Read the model definition and answer for the solid it produces. Units are mm, in the model's axes. A direction names the side the tool comes from. Coordinates: 2 decimals unless noted, no trailing zeros. Loops run counter-clockwise (first coordinate to the right, second up) from the corner with the lowest first, then second, coordinate; pieces in that order, holes last. Notation, with made-up numbers: M 21,65.5 L 59,65.5 A25 cw 59,91.5 Z; hole C 54,59 d3. An arc over 180 degrees is marked long. One line per item, written item: value. Start each with the question number.
1. Determine the mould class of faces 1 (the face through (-6, -29.725, -89)), 2 (the face through (-4, 30, -89)), 3 (the face through (-2, -35.725, -89)) for opening direction Y: +Y half, -Y half, draft (parallel to the pull), parting line (faces both ways), or undercut.
2. The part is cut by section A-A (z = -16). Write down the section's boundary in (x, y) (3 decimals).
3. Flat-ended cylindrical pins translate along their axes: pin 1 (1.5 mm diameter, centred on x = 6.5, z = -23, fed in from -Y) (3 decimals); pin 2 (1.2 mm diameter, centred on x = -5, z = -72.5, fed in from +Y) (3 decimals); pin 3 (6.5 mm diameter, centred on y = -26, z = -47.5, fed in from -X). Find the tip coordinate at first contact, or state that the pin passes through.
4. For faces 4 (the face through (-8, -33, -89)), 5 (the face through (8, 23.725, -89)), 6 (the face through (-4, -27, -89)), determine the directions among +Z, -Z, +X, -X, +Y, -Y from which every point of the face is accessible in a straight line to the end or side of a thin tool.
5. Consider probe 1 along Y at (x, z) = (4.25, -64.5) (3 decimals); probe 2 along Y at (x, z) = (-4.25, -117) (3 decimals); probe 3 along X at (y, z) = (-17, -14.5). Determine where each line is inside the solid, lowest interval first.
6. The part is cut by section B-B (y = 12.5). Write down the section's boundary in (x, z).
7. The part is cut by section C-C (y = -11.5). Write down the section's boundary in (x, z).
```python
from build123d import *

# Parameters (mm, degrees)
EXTRUDE_1_DEPTH = 180


with BuildPart() as part:
    # Эскиз1 → Бобышка-Вытянуть1 (new body)
    with BuildSketch(Plane.XY):
        with BuildLine():
            Line((-11, -23.725), (-4, -23.725))
            Line((-4, -23.725), (-4, -29.725))
            Line((-4, -29.725), (-8, -29.725))
            Line((-8, -29.725), (-8, -35.725))
            Line((-8, -35.725), (4, -35.725))
            Line((4, -35.725), (4, -23.725))
            Line((4, -23.725), (11, -23.725))
            ThreePointArc((11, -23.725), (5.012775134, 0), (11, 23.725))
            Line((11, 23.725), (4, 23.725))
            Line((4, 23.725), (4, 29.725))
            Line((4, 29.725), (8, 29.725))
            Line((8, 29.725), (8, 35.725))
            Line((8, 35.725), (-4, 35.725))
            Line((-4, 35.725), (-4, 23.725))
            Line((-4, 23.725), (-11, 23.725))
            ThreePointArc((-11, 23.725), (-5.012775134, 0), (-11, -23.725))
        make_face()
    extrude(amount=-EXTRUDE_1_DEPTH)


solid = part.part
```
Answer block:
1. face 1: undercut
1. face 2: draft
1. face 3: -Y half
2. outline: M -11,-23.725 L -4,-23.725 L -4,-29.725 L -8,-29.725 L -8,-35.725 L 4,-35.725 L 4,-23.725 L 11,-23.725 A50 cw 11,23.725 L 4,23.725 L 4,29.725 L 8,29.725 L 8,35.725 L -4,35.725 L -4,23.725 L -11,23.725 A50 cw Z
3. pin 1: stops at y = -23.725
3. pin 2: stops at y = 23.725
3. pin 3: stops at x = -11
4. face 4: +Z, -Z, -X, -Y
4. face 5: +Z, -Z, +X
4. face 6: +Z, -Z, -X
5. probe 1: y = -23.725 to 23.725, 29.725 to 35.725
5. probe 2: y = -35.725 to -29.725, -23.725 to 23.725
5. probe 3: x = -7.99 to 7.99
6. outline: M -6.6,-180 L 6.6,-180 L 6.6,0 L -6.6,0 Z
7. outline: M -6.35,-180 L 6.35,-180 L 6.35,0 L -6.35,0 Z
